Could you check a few things on this model? Use its own coordinates, in mm. A direction names the side the tool comes from. Give positions to 0.01 mm unless a question says otherwise; leave off trailing zeros. Loops run counter-clockwise (first coordinate to the right, second up) from the corner with the lowest first, then second, coordinate; pieces in that order, holes last. Notation, with made-up numbers: (16, 34) - (52, 34) arc R10 ccw to (52, 52) - close; hole circle Ø10 at (-1, 82.25). An arc over 180 degrees is marked (long way). Answer in a Markdown table with one row per item. Add a question column.
```python
from build123d import *

# Parameters (mm, degrees)
F1_DEPTH    = 12.7
F2_W        = 2.54
F2_H        = 7.62
F3_DEPTH    = 20.32
F4_R        = 1.27
F5_DEPTH    = 25.4
F6_R        = 1.27
F7_DEPTH    = 25.4
F8_T1_DEPTH = 24.0023585695
F8_T3_DEPTH = 24.0023585695
F8_T5_DEPTH = 24.0023585695
F8_T7_DEPTH = 24.0023585695


# Not quite as in the source:
# - a fillet or chamfer that OpenCascade refuses, or shapes differently, is made with other operations: its cross-section is extruded or revolved along the edge and cut away or added


with BuildPart() as f1:
    # F0 (on Front) → F1 (new body)
    with BuildSketch(Plane.XZ):
        Polygon((32.2204480681, 39.2744538637), (-50.1228987998, 8.2664996165), (17.9024507316, -47.5409534801), align=None)
    extrude(amount=F1_DEPTH)

    # F2 (on face) → F3 (join)
    with BuildSketch(Plane(origin=(-16.1102240341, 0, -19.6372269318), x_dir=(0.7731191705, 0, -0.6342607887), z_dir=(-0.6342607887, 0, -0.7731191705))):
        with Locations((-16.51, 6.3304389822)):
            Rectangle(F2_W, F2_H)
        with Locations((16.51, 6.3037265553)):
            Rectangle(F2_W, F2_H)
    extrude(amount=F3_DEPTH)

    # F4 (on face) → F5 (cut)
    with BuildSketch(Plane(origin=(-13.7460588523, 0, 11.2771568238), x_dir=(0, -1, 0), z_dir=(-0.7731191705, 0, 0.6342607887))):
        with Locations((6.3304389822, -39.37)):
            Circle(F4_R)
    extrude(amount=-F5_DEPTH, mode=Mode.SUBTRACT)

    # F6 (on face) → F7 (cut)
    with BuildSketch(Plane(origin=(11.7823361591, 0, -9.6661344204), x_dir=(0, -1, 0), z_dir=(-0.7731191705, 0, 0.6342607887))):
        with Locations((6.3037265553, -39.37)):
            Circle(F6_R)
    extrude(amount=-F7_DEPTH, mode=Mode.SUBTRACT)

    # F8: fillet of radius 4.2924717139 on 4 edges, made by hand

    # F8_s2 → F8_t1 (cut)
    with BuildSketch(Plane(origin=(-22.0425392799, 0, 18.0835230611), x_dir=(0, 1, 0), z_dir=(0.7731191705, 0, -0.6342607887))):
        with BuildLine():
            ThreePointArc((-2.5204389822, -41.4275282861), (-3.7776748391, -44.4627641431), (-6.8129106961, -45.72))
            Line((-6.8129106961, -45.72), (-2.5204389822, -45.72))
            Line((-2.5204389822, -45.72), (-2.5204389822, -41.4275282861))
        make_face()
    extrude(amount=F8_T1_DEPTH, mode=Mode.SUBTRACT)

    # F8_s4 → F8_t3 (cut)
    with BuildSketch(Plane(origin=(-3.4858557315, 0, 2.8597681832), x_dir=(0, 1, 0), z_dir=(-0.7731191705, 0, 0.6342607887))):
        with BuildLine():
            ThreePointArc((-10.1404389822, 41.4275282861), (-8.8832031252, 44.4627641431), (-5.8479672683, 45.72))
            Line((-5.8479672683, 45.72), (-10.1404389822, 45.72))
            Line((-10.1404389822, 45.72), (-10.1404389822, 41.4275282861))
        make_face()
    extrude(amount=F8_T3_DEPTH, mode=Mode.SUBTRACT)

    # F8_s6 → F8_t5 (cut)
    with BuildSketch(Plane(origin=(3.4858557315, 0, -2.8597681832), x_dir=(0, 1, 0), z_dir=(0.7731191705, 0, -0.6342607887))):
        with BuildLine():
            ThreePointArc((-2.4937265553, -41.4275282861), (-3.7509624122, -44.4627641431), (-6.7861982692, -45.72))
            Line((-6.7861982692, -45.72), (-2.4937265553, -45.72))
            Line((-2.4937265553, -45.72), (-2.4937265553, -41.4275282861))
        make_face()
    extrude(amount=F8_T5_DEPTH, mode=Mode.SUBTRACT)

    # F8_s8 → F8_t7 (cut)
    with BuildSketch(Plane(origin=(22.0425392799, 0, -18.0835230611), x_dir=(0, 1, 0), z_dir=(-0.7731191705, 0, 0.6342607887))):
        with BuildLine():
            ThreePointArc((-10.1137265553, 41.4275282861), (-8.8564906983, 44.4627641431), (-5.8212548414, 45.72))
            Line((-5.8212548414, 45.72), (-10.1137265553, 45.72))
            Line((-10.1137265553, 45.72), (-10.1137265553, 41.4275282861))
        make_face()
    extrude(amount=F8_T7_DEPTH, mode=Mode.SUBTRACT)


solid = f1.part
```
(1) I want a section at A-A on y = -1. Please give me the cut outline in (x, z).
(2) For pin 1 Ø3.5 at (x, z) = (-8, -34) entering from -Y; pin 2 Ø3 at (x, y) = (-24, -9.5) entering from +Z; pin 3 Ø6 at (x, z) = (-6.5, -38.5) entering from +Y; pin 4 Ø2 at (x, z) = (-39.5, -16) entering from +Y, each with a flat end and sliding along its axis, tell me the tip position at first contact or that it passes through.
(3) We'd pull the mould along X, two halves only. Please class faces 4 (the cylindrical face through (-15.29, -9.05, -44.7)), 5 (the cylindrical face through (-38.057, -7.504, -20.331)), 6 (the flat face through (-8, -10.114, -36)): pulls with the +X half, pulls with the -X half, needs draft (parallel to the pull), parting line crosses it, or undercut.
(4) I want a section at B-B on z = -3. Please give me the cut outline in (x, y), then the cut area to 3 significant figures.
(5) Please list where these lines run through material, in increasing order: line 1 (X direction, y = -4.25, z = -31); line 2 (X direction, y = -8.5, z = -39); line 3 (Z direction, x = -2, y = -2.5).
(6) I want a section at C-C on x = -20.5. Please give me the cut outline in (y, z).
(7) On a 3-axis mill with a long thin cutter (end or side, diameter ignored), from which of +Z, -Z, +X, -X, +Y, -Y can I reach the whole of each face in a straight line? I mean faces 1 (the flat face through (-34, -2.52, -15)), 2 (the flat face through (-34, -10.14, -15)), 3 (the flat face through (-34.24, -6.28, -17.71)). Say none if no direction works.
Reported:
| question | item | result |
|---|---|---|
| 1 | outline | (-50.12, 8.27) - (17.9, -47.54) - (32.22, 39.27) - close |
| 2 | pin 1 | y = -10.11 |
| 2 | pin 2 | z = 18.67 |
| 2 | pin 3 | y = -2.49 |
| 2 | pin 4 | through |
| 3 | face 4 | pulls with the -X half |
| 3 | face 5 | undercut |
| 3 | face 6 | needs draft |
| 4 | outline | (-36.39, -12.7) - (25.25, -12.7) - (25.25, 0) - (-36.39, 0) - close |
| 4 | area | 783 mm² |
| 5 | line 1 | -5.72 to -2.43, -2.26 to 20.63 |
| 5 | line 2 | -12.28 to -9, 7.49 to 19.31 |
| 5 | line 3 | -31.21 to 26.39 |
| 6 | outline | (-12.7, -16.04) - (0, -16.04) - (0, 19.42) - (-12.7, 19.42) - close |
| 7 | face 1 | -Z, -X, +Y |
| 7 | face 2 | -Z, -X, -Y |
| 7 | face 3 | -Z, +Y, -Y |
